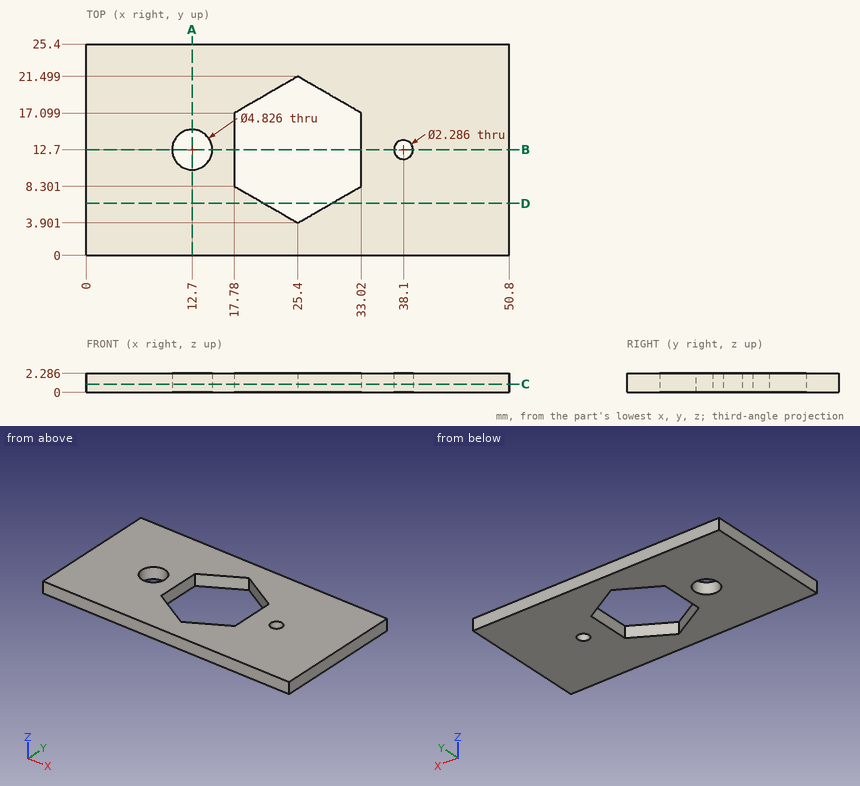
For this review, use the dimensioned drawing (mm, ordinates from the lowest corner) and the shaded views. Give positions to 0.01 mm unless a question says otherwise; leave off trailing zeros. Loops run counter-clockwise (first coordinate to the right, second up) from the corner with the lowest first, then second, coordinate; pieces in that order, holes last.
Item 1: For line 1 along Y through (x, z) = (38.1, 0.8); line 2 along Y through (x, z) = (12.7, 0.95); line 3 along X through (y, z) = (16.5, 0.9), list the stretches that pass through material, from the lowest coordinate up.
Item 2: Take a section at C-C, the plane z = 1. State the section outline as (x, y) points.
Item 3: Take a section at A-A, the plane x = 12.7. State the section outline as (y, z) points.
Item 4: Insertion check: pin 1 (1.4 mm diameter, centred on x = 38.1, y = 12.7, fed in from -Z). The pin has a flat end and moves straight along its axis. Give the tip position at first contact, or say it passes through.
Item 5: Take a section at D-D, the plane y = 6.25. State the section outline as (x, z) points.
Item 6: Take a section at B-B, the plane y = 12.7. State the section outline as (x, z) points.
Calculated:
1. line 1: y = 0 to 11.56, 13.84 to 25.4
1. line 2: y = 0 to 10.29, 15.11 to 25.4
1. line 3: x = 0 to 17.78, 33.02 to 50.8
2. outline: (0, 0) - (50.8, 0) - (50.8, 25.4) - (0, 25.4) - close; hole circle Ø4.83 at (12.7, 12.7); hole (17.78, 8.3) - (25.4, 3.9) - (33.02, 8.3) - (33.02, 17.1) - (25.4, 21.5) - (17.78, 17.1) - close; hole circle Ø2.29 at (38.1, 12.7)
3. outline: (0, 0) - (10.29, 0) - (10.29, 2.29) - (0, 2.29) - close; (15.11, 0) - (25.4, 0) - (25.4, 2.29) - (15.11, 2.29) - close
4. pin 1: passes through
5. outline: (0, 0) - (21.33, 0) - (21.33, 2.29) - (0, 2.29) - close; (29.47, 0) - (50.8, 0) - (50.8, 2.29) - (29.47, 2.29) - close
6. outline: (0, 0) - (10.29, 0) - (10.29, 2.29) - (0, 2.29) - close; (15.11, 0) - (17.78, 0) - (17.78, 2.29) - (15.11, 2.29) - close; (33.02, 0) - (36.96, 0) - (36.96, 2.29) - (33.02, 2.29) - close; (39.24, 0) - (50.8, 0) - (50.8, 2.29) - (39.24, 2.29) - close
